Could you check a few things on this model? Use its own coordinates, in mm. A direction names the side the tool comes from. Round coordinates to 2 decimals unless told otherwise and drop trailing zeros. Loops run counter-clockwise (first coordinate to the right, second up) from the corner with the lowest first, then second, coordinate; pieces in that order, holes last. Notation, with made-up numbers: (-22, 77.5) -> (16, 77.5) arc R26 cw to (16, 110.5) -> close; hole circle Ø2 at (15.25, -17). An arc over 180 degrees is marked (long way). One line per item, written item: value.
Autodesk Inventor part; units mm, degrees
ref_plane "YZ Plane" through (0, 0, 0) normal (1, 0, 0) x (0, 1, 0)
ref_plane "XZ Plane" through (0, 0, 0) normal (0, 1, 0) x (-1, 0, 0)
ref_plane "XY Plane" through (0, 0, 0) normal (0, 0, 1) x (1, 0, 0)
sketch "Эскиз1" plane through (0, 0, 0) normal (0, 1, 0) x (-1, 0, 0)
  line L0 (-8.725, 50) -> (8.725, 50)
  line L1 (8.725, 50) -> (8.725, -50)
  line L2 (8.725, -50) -> (-8.725, -50)
  line L3 (-8.725, -50) -> (-8.725, 50)
  line L4 (-8.725, 50) -> (8.725, -50) construction
  line L5 (8.725, 50) -> (-8.725, -50) construction
  line L6 (-8.725, 50) -> (0.475, 50)
  line L7 (0.475, 50) -> (0.475, 47.05)
  line L8 (0.475, 47.05) -> (-8.725, 47.05)
  line L9 (-8.725, 47.05) -> (-8.725, 50)
  point P0 (0, 0)
  point P1 (0.475, 50)
  dimension "d0" = 17.45
  dimension "d1" = 100
  dimension "d13" = 9.2
  dimension "d14" = 2.95
extrude "Выдавливание1" add sketch "Эскиз1" along normal blind 3 contours L0 L1 L2 L3 L8 L7
mirror "Зеркальное отражение1" about plane through (-8.725, 0, -50) normal (-1, 0, 0)
sketch "Эскиз2" plane through (0, 3, 0) normal (0, 1, 0) x (1, 0, 0)
  line L0 (-8.725, -50) -> (-8.725, -39.05) construction
  line L1 (-21.175, -39.05) -> (3.725, -39.05)
  line L2 (-0.475, -50) -> (-16.975, -50)
  line L3 (-21.725, 47.2) -> (4.275, 47.2)
  line L4 (-21.725, 26) -> (4.275, 26)
  line L5 (-8.725, 26) -> (-8.725, 47.2)
  line L6 (-8.725, 47.2) -> (-8.725, 50)
  line L7 (8.725, 50) -> (-26.175, 50)
  dimension "d4" = 10.95
  dimension "d5" = 24.9
  dimension "d15" = 26
  dimension "d16" = 2.8
  dimension "d17" = 21.2
hole "Отверстие1" at (3.725, 3, 39.05) at (-21.175, 3, 39.05) at (-21.725, 3, -26) at (4.275, 3, -26) at (4.275, 3, -47.2) at (-21.725, 3, -47.2) direction (0, -1, 0) diameter 3.2 end through all
properties part number "Basis of the robot"
(1) If I drill on L1, parallel to X at y = 2.25, z = 39.05 (3 decimals); L2, parallel to X at y = 2.25, z = -47.2 (3 decimals); L3, parallel to Z at x = -23, y = 0.2, over which ranges is the centre line in solid material (lowest first)?
Recorded:
L1: -26.175 to -22.775, -19.575 to 2.125, 5.325 to 8.725
L2: -26.175 to -23.325, -20.125 to 2.675, 5.875 to 8.725
L3: -50 to -48.17, -46.23 to -26.97, -25.03 to 47.05
(2) If we section it at B-B, the plane y = 1.1: Please give me the cut outline in (x, z) (3 decimals), then the cut area to 3 significant figures.
Recorded:
outline: (-26.175, -50) -> (8.725, -50) -> (8.725, 47.05) -> (-0.475, 47.05) -> (-0.475, 50) -> (-16.975, 50) -> (-16.975, 47.05) -> (-26.175, 47.05) -> close; hole circle Ø3.2 at (-21.725, -47.2); hole circle Ø3.2 at (-21.725, -26); hole circle Ø3.2 at (-21.175, 39.05); hole circle Ø3.2 at (3.725, 39.05); hole circle Ø3.2 at (4.275, -47.2); hole circle Ø3.2 at (4.275, -26)
area: 3,390 mm²
(3) If we section it at A-A, the plane z = -47.2: Please give me the cut outline in (x, y) (3 decimals).
Recorded:
outline: (-26.175, 0) -> (-23.325, 0) -> (-23.325, 3) -> (-26.175, 3) -> close; (-20.125, 0) -> (2.675, 0) -> (2.675, 3) -> (-20.125, 3) -> close; (5.875, 0) -> (8.725, 0) -> (8.725, 3) -> (5.875, 3) -> close
(4) I'm going to push flat-ended pins straight in: pin 1 Ø0.9 at (y, z) = (2, 48.5) entering from -X (3 decimals); pin 2 Ø4 at (x, z) = (4.275, -26) entering from +Y; pin 3 Ø0.9 at (x, y) = (-21, 2) entering from +Z. Where does each tip first touch, or does it pass through?
Recorded:
pin 1: x = -16.975
pin 2: y = 3
pin 3: z = 47.05
(5) For faces 4 (the face through (-22, 1, 47.05)), 5 (the face through (-0.475, 1, 49)), 6 (the face through (-9, 1, 50)), which set-ups out of +Z, -Z, +X, -X, +Y, -Y let a thin tool reach every point of the face, with its end or its side?
Recorded:
face 4: +Z, -X, +Y, -Y
face 5: +Z, +X, +Y, -Y
face 6: +Z, +X, -X, +Y, -Y
(6) Thinking about a two-plate mould opening in Z: for faces 1 (the face through (-22.206, 1.479, -45.674)), 2 (the face through (8.725, 1, -2)), 3 (the face through (4, 1, 47.05)), which applies, released by +Z, released by -Z, zero draft, split by the parting line, or undercut?
Recorded:
face 1: undercut
face 2: zero draft
face 3: released by +Z
